Input: dimensioned drawing with shaded views. Units: mm. Origin: part minimum x, y, z. A direction names the side the tool comes from. Round coordinates to 2 decimals unless told otherwise and drop trailing zeros. Loops run counter-clockwise (first coordinate to the right, second up) from the corner with the lowest first, then second, coordinate; pieces in that order, holes last. Notation, with made-up numbers: (-6, 41.25) - (46, 41.25) arc R15 ccw to (46, 49.25) - close; hole circle Ø8 at (36, 76.25). An arc over 180 degrees is marked (long way). Write each question's results on one line, items separated by ' | '.
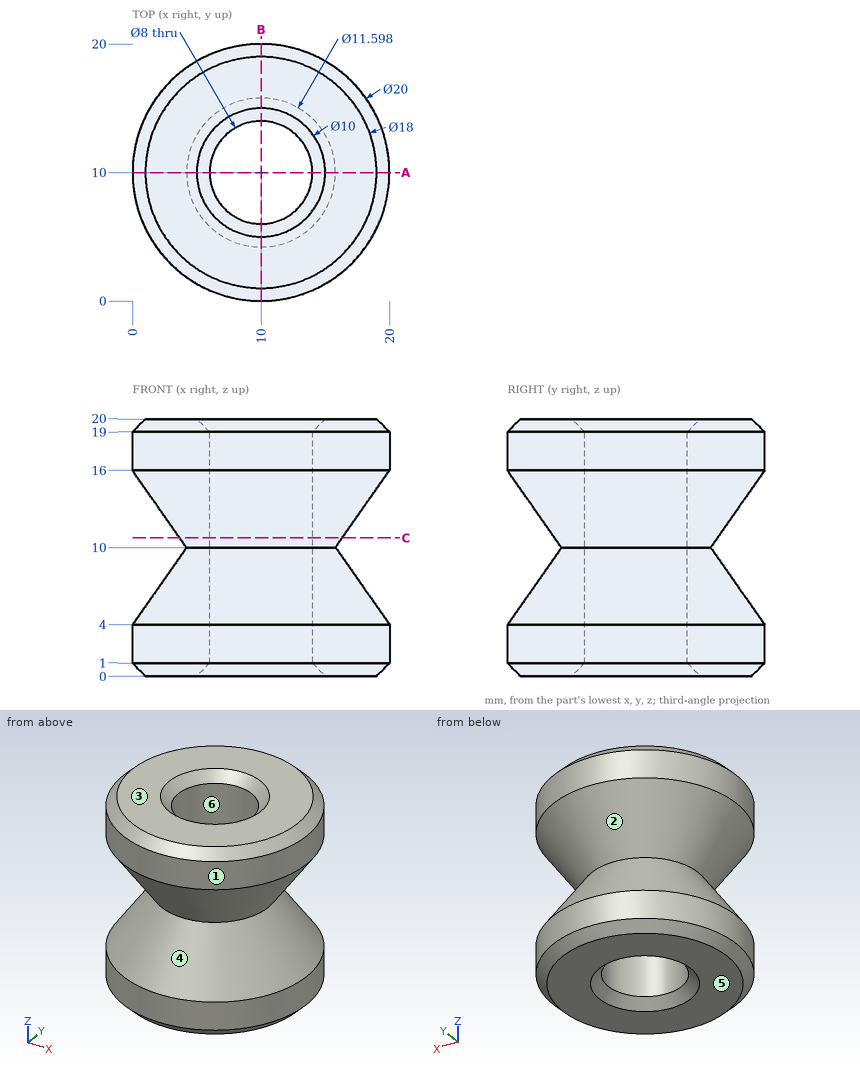
1. Section query A-A, the plane y = 10. Output: boundary loops of the cut face in (x, z).
Answer:
outline: (0, 1) - (1, 0) - (5, 0) - (6, 1) - (6, 19) - (5, 20) - (1, 20) - (0, 19) - (0, 16) - (4.2, 10) - (0, 4) - close; (14, 1) - (15, 0) - (19, 0) - (20, 1) - (20, 4) - (15.8, 10) - (20, 16) - (20, 19) - (19, 20) - (15, 20) - (14, 19) - close
2. Set-up query: the marked faces 1 and 2. Return all of +Z, -Z, +X, -X, +Y, -Y with unobstructed straight access to the full face (end or side cutting, diameter ignored); none if empty.
Answer:
face 1: +Z, -Z | face 2: none
3. Line query: line 1 (Z direction, x = 9.5, y = 17); line 2 (Z direction, x = 15, y = 4) (1 decimal); line 3 (X direction, y = 10.25, z = 13.75). Output: solid intervals per line, ascending. Write a range as [from, to].
Answer:
line 1: [0, 8.26], [11.74, 20] | line 2: [0, 7.1], [12.9, 20] | line 3: [1.58, 6.01], [13.99, 18.42]
4. Mould query, pull axis Z, two halves, no side actions, for the marked faces 3, 4, 5 and 6. Classes: pulls with the +Z half, pulls with the -Z half, needs draft (parallel to the pull), parting line crosses it, or undercut.
Answer:
face 3: pulls with the +Z half | face 4: undercut | face 5: pulls with the -Z half | face 6: needs draft
5. Section query C-C, the plane z = 10.75. Output: boundary loops of the cut face in (x, y).
Answer:
outline: circle Ø12.65 at (10, 10); hole circle Ø8 at (10, 10)
6. Contact query for flat-ended pins moving along their axis: pin 1 (8 mm diameter, centred on y = 9, z = 8.5, fed in from -X); pin 2 (4 mm diameter, centred on x = 7.5, y = 11, fed in from -Z); pin 3 (8 mm diameter, centred on x = 17, z = 3, fed in from -Y); pin 4 (7 mm diameter, centred on x = 10, y = 10, fed in from -Z). Output: stop coordinate, or through.
Answer:
pin 1: x = 0.38 | pin 2: z = 0.31 | pin 3: y = 0.46 | pin 4: through
